Here's how the part is built. I have some questions about the finished solid (model axes, mm). Round coordinates to 2 decimals unless told otherwise and drop trailing zeros. Write each loop counter-clockwise with the first axis right and the second up, starting at its lowest first coordinate (ties: lowest second). Pieces come first, ordered by that corner, then holes. Notation, with made-up numbers: (69.5, -4.5) -> (106.5, -4.5) arc R14 ccw to (106.5, 18.5) -> close; hole circle Ø11 at (8, 3.25). An arc over 180 degrees is marked (long way). Answer as CSV lines item,"result".
from build123d import *

# Parameters (mm, degrees)
CROQUIS1_R              = 3
CROQUIS1_R_2            = 11.5
CROQUIS1_R_3            = 12.5
SALIENTE_EXTRUIR1_DEPTH = 5


with BuildPart() as part:
    # Croquis1 → Saliente-Extruir1 (new body)
    with BuildSketch(Plane(origin=(0, 0, 0), x_dir=(1, 0, 0), z_dir=(0, 1, 0))):
        Polygon((-158.326848249, 165.982121671), (231.673151751, 165.982121671), (231.673151751, 135.982121671), (261.673151751, 135.982121671), (261.673151751, -204.017878329), (231.673151751, -204.017878329), (231.673151751, -234.017878329), (-158.326848249, -234.017878329), (-158.326848249, -204.017878329), (-188.326848249, -204.017878329), (-188.326848249, 135.982121671), (-158.326848249, 135.982121671), align=None)
        with Locations(Location((-173.326848249, 35.982121671, 0), (0, 0, 270))):
            Circle(CROQUIS1_R, mode=Mode.SUBTRACT)
        with Locations(Location((-173.326848249, -104.017878329, 0), (0, 0, 270))):
            Circle(CROQUIS1_R, mode=Mode.SUBTRACT)
        with Locations(Location((-48.326848249, 150.982121671, 0), (0, 0, 270))):
            Circle(CROQUIS1_R, mode=Mode.SUBTRACT)
        with Locations(Location((121.673151751, 150.982121671, 0), (0, 0, 270))):
            Circle(CROQUIS1_R, mode=Mode.SUBTRACT)
        with Locations(Location((246.673151751, 35.982121671, 0), (0, 0, 270))):
            Circle(CROQUIS1_R, mode=Mode.SUBTRACT)
        with Locations(Location((246.673151751, -104.017878329, 0), (0, 0, 270))):
            Circle(CROQUIS1_R, mode=Mode.SUBTRACT)
        with Locations(Location((-48.326848249, -219.017878329, 0), (0, 0, 270))):
            Circle(CROQUIS1_R, mode=Mode.SUBTRACT)
        with Locations(Location((121.673151751, -219.017878329, 0), (0, 0, 270))):
            Circle(CROQUIS1_R, mode=Mode.SUBTRACT)
        with Locations(Location((-135.826848249, -64.017878329, 0), (0, 0, 270))):
            Circle(CROQUIS1_R_2, mode=Mode.SUBTRACT)
        with Locations(Location((-135.826848249, -114.017878329, 0), (0, 0, 270))):
            Circle(CROQUIS1_R_3, mode=Mode.SUBTRACT)
        with Locations(Location((-135.826848249, -14.017878329, 0), (0, 0, 270))):
            Circle(CROQUIS1_R_3, mode=Mode.SUBTRACT)
        with Locations(Location((209.173151751, -114.017878329, 0), (0, 0, 90))):
            Circle(CROQUIS1_R_3, mode=Mode.SUBTRACT)
        with Locations(Location((209.173151751, -64.017878329, 0), (0, 0, 90))):
            Circle(CROQUIS1_R_2, mode=Mode.SUBTRACT)
        with Locations(Location((209.173151751, -14.017878329, 0), (0, 0, 90))):
            Circle(CROQUIS1_R_3, mode=Mode.SUBTRACT)
    extrude(amount=SALIENTE_EXTRUIR1_DEPTH)


solid = part.part
Item 1: Suppose I cut it at A-A, the plane y = 3.3. State how many separate pieces and enclosed holes the cut face has, then the cut area to 3 significant figures.
Results found:
separate pieces,"1"
enclosed holes,"14"
area,"173,000 mm²"
Item 2: I need wall thicknesses on L1, parallel to X at y = 0.65, z = 74; L2, parallel to X at y = 3.45, z = -143; L3, parallel to Z at x = -138, y = 3.65. Which ranges of each line are inside material? Lowest first, please.
Results found:
L1,"x = -188.33 to -141.54, -130.12 to 203.46, 214.88 to 261.67"
L2,"x = -158.33 to 231.67"
L3,"z = -165.98 to 1.71, 26.33 to 52.73, 75.31 to 101.71, 126.33 to 234.02"
Item 3: Suppose I cut it at B-B, the plane z = 57.5. List the corners of the cut face in (x, y) for me.
Results found:
outline,"(-188.33, 0) -> (-145.3, 0) -> (-145.3, 5) -> (-188.33, 5) -> close; (-126.35, 0) -> (199.7, 0) -> (199.7, 5) -> (-126.35, 5) -> close; (218.65, 0) -> (261.67, 0) -> (261.67, 5) -> (218.65, 5) -> close"
Item 4: If we mould it in two halves opening along Z, with no side actions, what happens to faces 1 (the flat face through (40, 5, 31)), 2 (the cylindrical face through (200.725, 2.465, 123.231)), 3 (the cylindrical face through (-123.433, 2.465, 12.391))? For each: pulls with the +Z half, pulls with the -Z half, needs draft (parallel to the pull), parting line crosses it, or undercut.
Results found:
face 1,"needs draft"
face 2,"undercut"
face 3,"undercut"
Item 5: Suppose I cut it at C-C, the plane z = -141. List the corners of the cut face in (x, y) for me.
Results found:
outline,"(-158.33, 0) -> (231.67, 0) -> (231.67, 5) -> (-158.33, 5) -> close"
Item 6: Will these pins go through, and if not, where does the flat tip stop? pin 1 (1.5 mm diameter, centred on x = -171.5, y = 2.5, fed in from -Z); pin 2 (4 mm diameter, centred on x = -15, z = 5.5, fed in from -Y); pin 3 (1.5 mm diameter, centred on y = 3.5, z = -144.5, fed in from -X); pin 4 (1.5 mm diameter, centred on y = 2, z = -151, fed in from +X).
Results found:
pin 1,"stops at z = -135.98"
pin 2,"stops at y = 0"
pin 3,"stops at x = -158.33"
pin 4,"stops at x = 231.67"
